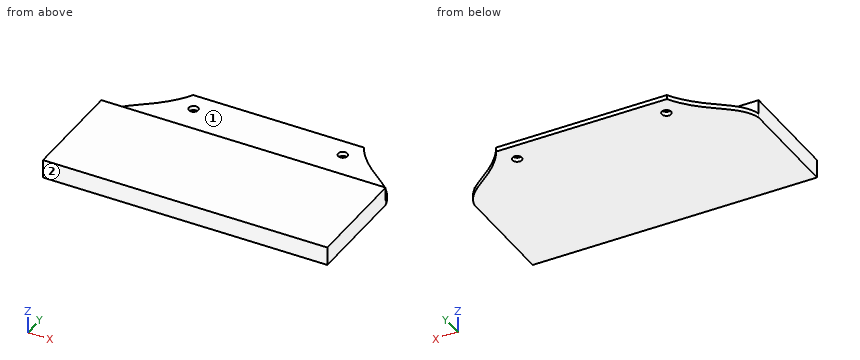
from build123d import *

# Parameters (mm, degrees)
F0_W     = 120
F0_H     = 45
F0_H_2   = 75
F0_W_2   = 40
F1_DEPTH = 3
F2_W     = 200
F2_H     = 75
F3_DEPTH = 10
F4_R     = 3.25
F5_DEPTH = 25


with BuildPart() as f1:
    # F0 (on Top) → F1 (new body)
    with BuildSketch(Plane.XY):
        Rectangle(F0_W, F0_H)
        with BuildLine():
            Line((-100, -22.5), (-60, -22.5))
            Line((-60, -22.5), (-60, 22.5))
            add(Edge.make_bspline(
                [(-100, -22.5), (-95.680383, -4.419341), (-73.623309, -1.538), (-60, 22.5)],
                knots=[0, 0, 0, 0, 60.207973, 60.207973, 60.207973, 60.207973], degree=3))
        make_face()
        with Locations((0, -60)):
            Rectangle(F0_W, F0_H_2)
        with Locations((-80, -60)):
            Rectangle(F0_W_2, F0_H_2)
        with Locations((80, -60)):
            Rectangle(F0_W_2, F0_H_2)
        with BuildLine():
            Line((60, 22.5), (60, -22.5))
            Line((60, -22.5), (100, -22.5))
            add(Edge.make_bspline(
                [(100, -22.5), (95.680383, -4.419341), (73.623309, -1.538), (60, 22.5)],
                knots=[0, 0, 0, 0, 60.207973, 60.207973, 60.207973, 60.207973], degree=3))
        make_face()
    extrude(amount=F1_DEPTH)

    # F2 (on face) → F3 (join)
    with BuildSketch(Plane.XY.offset(3)):
        with Locations((0, -60)):
            Rectangle(F2_W, F2_H)
    extrude(amount=F3_DEPTH)

    # F4 (on face) → F5 (cut)
    with BuildSketch(Plane.XY.offset(3)):
        with Locations((-52.5, 9.25)):
            Circle(F4_R)
        with Locations((52.5, 9.25)):
            Circle(F4_R)
    extrude(amount=-F5_DEPTH, mode=Mode.SUBTRACT)


solid = f1.part
The listing builds one solid part. Answer for the finished solid, in the listing's coordinates (mm). Face numbers are marked on the shaded views. A direction names the side the tool comes from. Coordinates: 2 decimals unless noted, no trailing zeros. Loops run counter-clockwise (first coordinate to the right, second up) from the corner with the lowest first, then second, coordinate; pieces in that order, holes last. Notation, with made-up numbers: M 10.25,-3.5 L 14.25,-3.5 A17 cw 14.25,25.5 Z; hole C 76.5,-19.5 d6. An arc over 180 degrees is marked long. Answer in a Markdown table with one row per item.
1) Find the intervals of material crossed by probe 1 along Y at (x, z) = (52.5, 1.4); probe 2 along Y at (x, z) = (89, 4.75); probe 3 along Z at (x, y) = (-63, -4), in increasing order.
Answers below:
| item | result |
|---|---|
| probe 1 | -97.5 to 6, 12.5 to 22.5 |
| probe 2 | -97.5 to -22.5 |
| probe 3 | 0 to 3 |
2) Which of the six approach directions +Z, -Z, +X, -X, +Y, -Y give full straight-line access (tool end or side, diameter ignored) to the marked faces 1 and 2?
Answers below:
| item | result |
|---|---|
| face 1 | +Z, +X, -X, +Y |
| face 2 | +Z, -Z, +X, -X, -Y |
3) Find section D-D (y = 9.25). Count the separate pieces of the cut face and the enclosed holes in it, then the cut area to 3 significant figures.
Answers below:
| item | result |
|---|---|
| separate pieces | 3 |
| enclosed holes | 0 |
| area | 381 mm^2 |
4) Find section A-A (x = 52.5). Determine the outline of the cut face in (y, z), then the cut area to 3 significant figures.
Answers below:
| item | result |
|---|---|
| outline | M -97.5,0 L 6,0 L 6,3 L -22.5,3 L -22.5,13 L -97.5,13 Z; M 12.5,0 L 22.5,0 L 22.5,3 L 12.5,3 Z |
| area | 1,090 mm^2 |
5) Find section B-B (x = -33). Determine the outline of the cut face in (y, z).
Answers below:
| item | result |
|---|---|
| outline | M -97.5,0 L 22.5,0 L 22.5,3 L -22.5,3 L -22.5,13 L -97.5,13 Z |
6) Given pin 1 (13.5 mm diameter, centred on x = -15.5, y = 4, fed in from +Z); pin 2 (3 mm diameter, centred on y = 5.5, z = 3, fed in from +X); pin 3 (8 mm diameter, centred on x = -28.5, y = -82.5, fed in from -Z), each flat-ended and moving along its own axis, determine where each tip first touches the part or whether it passes through.
Answers below:
| item | result |
|---|---|
| pin 1 | z = 3 |
| pin 2 | x = 75.66 |
| pin 3 | z = 0 |
7) Find section C-C (z = 7). Determine the outline of the cut face in (x, y), then the cut area to 3 significant figures.
Answers below:
| item | result |
|---|---|
| outline | M -100,-97.5 L 100,-97.5 L 100,-22.5 L -100,-22.5 Z |
| area | 15,000 mm^2 |
